Part model, mm, in its own coordinate system. A direction names the side the tool comes from. Round coordinates to 2 decimals unless told otherwise and drop trailing zeros. Write each loop counter-clockwise with the first axis right and the second up, starting at its lowest first coordinate (ties: lowest second). Pieces come first, ordered by that corner, then holes.
1) Flat gauge pins, fed straight in: pin 1 (1 mm diameter, centred on x = -42.5, z = 7.5, fed in from -Y); pin 2 (1.5 mm diameter, centred on x = 17.5, y = -7.5, fed in from +Z). Where does each tip first touch, or does it go through?
2) Pull direction X, two halves, no side cores. Call faces 1 (the cylindrical face through (48.041, 26.643, 8.409)), 2 (the cylindrical face through (49.991, -28.935, 7.395)), 3 (the flat face through (-1, 0, 0)): +X half, -X half, draft (parallel to the pull), parting line (faces both ways), or undercut.
3) Saw through at A-A on z = 8. Count the separate pieces of the cut face and the enclosed holes in it, and give its area (3 significant figures).
4) Saw through at D-D on x = -26. Write the cut outline in (y, z), and give its area (3 significant figures).
5) Saw through at B-B on x = 0. Write the cut outline in (y, z), and give its area (3 significant figures).
6) Saw through at C-C on y = 0. Write the cut outline in (x, z), and give its area (3 significant figures).
7) Drill centre lines: L1, parallel to X at y = 6, z = 10.75; L2, parallel to Z at x = 52.4, y = 0; L3, parallel to Y at x = -13, z = 8. Where is each one in solid material? Low to high.
8) Which spindle directions (+Z, -Z, +X, -X, +Y, -Y) get a long thin tool onto all of the face, cutting with end or side? Do faces 4 (the flat face through (-1, 0, 2)), 5 (the cylindrical face through (52.229, 0.325, 6.536)). Say none if no direction does.
```python
from build123d import *

# Parameters (mm, degrees)
PAD001_DEPTH       = 2
PAD003_DEPTH       = 15
SKETCH_R           = 1.5
POCKET_DEPTH       = 285.532619
POLARPATTERN_COUNT = 4


with BuildPart() as part:
    # Sketch001 → Pad001 (new body)
    with BuildSketch(Plane.XY):
        with BuildLine():
            Line((-53.75, 20), (-53.75, -20))
            ThreePointArc((-53.75, -20), (-50.088835, -28.838835), (-41.25, -32.5))
            Line((-41.25, -32.5), (41.25, -32.5))
            ThreePointArc((41.25, -32.5), (50.088835, -28.838835), (53.75, -20))
            Line((53.75, -20), (53.75, 20))
            ThreePointArc((53.75, 20), (50.088835, 28.838835), (41.25, 32.5))
            Line((41.25, 32.5), (-41.25, 32.5))
            ThreePointArc((-41.25, 32.5), (-50.088835, 28.838835), (-53.75, 20))
        make_face()
    extrude(amount=PAD001_DEPTH)

    # Sketch003 → Pad003 (join)
    with BuildSketch(Plane.XY):
        with BuildLine():
            Line((-41.25, 32.5), (41.25, 32.5))
            ThreePointArc((53.75, 20), (50.088835, 28.838835), (41.25, 32.5))
            Line((53.75, 20), (53.75, -20))
            ThreePointArc((41.25, -32.5), (50.088835, -28.838835), (53.75, -20))
            Line((41.25, -32.5), (-41.25, -32.5))
            ThreePointArc((-53.75, -20), (-50.088835, -28.838835), (-41.25, -32.5))
            Line((-53.75, -20), (-53.75, 20))
            ThreePointArc((-41.25, 32.5), (-50.088835, 28.838835), (-53.75, 20))
        make_face()
        with BuildLine():
            Line((-50.75, 20), (-50.75, -20))
            ThreePointArc((-50.75, -20), (-47.967514, -26.717514), (-41.25, -29.5))
            Line((-41.25, -29.5), (41.25, -29.5))
            ThreePointArc((41.25, -29.5), (47.967514, -26.717514), (50.75, -20))
            Line((50.75, -20), (50.75, 20))
            ThreePointArc((50.75, 20), (47.967514, 26.717514), (41.25, 29.5))
            Line((41.25, 29.5), (-41.25, 29.5))
            ThreePointArc((-41.25, 29.5), (-47.967514, 26.717514), (-50.75, 20))
        make_face(mode=Mode.SUBTRACT)
    extrude(amount=PAD003_DEPTH)

    # Sketch → Pocket (cut, through all)
    with BuildSketch(Plane.XZ):
        with Locations((0, 8)):
            Circle(SKETCH_R)
    pocket = extrude(amount=-POCKET_DEPTH, mode=Mode.SUBTRACT)

    # PolarPattern: Pocket ×4 about axis
    polarpattern_axis = Axis((0, 0, 0), (0, 0, 1))
    for i in range(1, POLARPATTERN_COUNT):
        add(pocket.rotate(polarpattern_axis, i * 360 / POLARPATTERN_COUNT), mode=Mode.SUBTRACT)


solid = part.part
```
Completed:
1. pin 1: stops at y = -32.48
1. pin 2: stops at z = 2
2. face 1: undercut
2. face 2: +X half
2. face 3: draft
3. separate pieces: 4
3. enclosed holes: 0
3. area: 906 mm2
4. outline: (-32.5, 0) - (32.5, 0) - (32.5, 15) - (29.5, 15) - (29.5, 2) - (-29.5, 2) - (-29.5, 15) - (-32.5, 15) - close
4. area: 208 mm2
5. outline: (-32.5, 0) - (32.5, 0) - (32.5, 6.5) - (29.5, 6.5) - (29.5, 2) - (-29.5, 2) - (-29.5, 6.5) - (-32.5, 6.5) - close; (-32.5, 9.5) - (-29.5, 9.5) - (-29.5, 15) - (-32.5, 15) - close; (29.5, 9.5) - (32.5, 9.5) - (32.5, 15) - (29.5, 15) - close
5. area: 190 mm2
6. outline: (-53.75, 0) - (53.75, 0) - (53.75, 6.5) - (50.75, 6.5) - (50.75, 2) - (-50.75, 2) - (-50.75, 6.5) - (-53.75, 6.5) - close; (-53.75, 9.5) - (-50.75, 9.5) - (-50.75, 15) - (-53.75, 15) - close; (50.75, 9.5) - (53.75, 9.5) - (53.75, 15) - (50.75, 15) - close
6. area: 275 mm2
7. L1: x = -53.75 to -50.75, 50.75 to 53.75
7. L2: z = 0 to 6.5, 9.5 to 15
7. L3: y = -32.5 to -29.5, 29.5 to 32.5
8. face 4: +Z
8. face 5: +X, -X
